Input: dimensioned drawing with shaded views. Units: mm. Origin: part minimum x, y, z. Round coordinates to 2 decimals unless told otherwise and drop trailing zeros. Order: outer loops, then holes, each group sorted by start corner. A loop starts at its lowest first (then second) coordinate and runs counter-clockwise, first axis right, second up.
Item 1: Cut plane B-B on y = 23. Output: boundary loops of the cut face in (x, z).
Item 2: Cut plane A-A on x = 13. Output: boundary loops of the cut face in (y, z), then the cut area to 3 significant figures.
Item 3: Cut plane C-C on z = 2.95. Output: boundary loops of the cut face in (x, y), then the cut area to 3 significant figures.
Item 4: Line query: L1, parallel to Y at x = 13, z = 2.85; L2, parallel to Y at x = 5, z = 3.2; L3, parallel to X at y = 16, z = 2.6. Output: solid intervals per line, ascending.
Item 5: First-contact query: pin 1 (4 mm diameter, centred on x = 21, y = 15, fed in from +Z); pin 2 (1.9 mm diameter, centred on x = 13, y = 23, fed in from -Z). Flat tips, straight axial feed; report the tip coordinate or a pass-through.
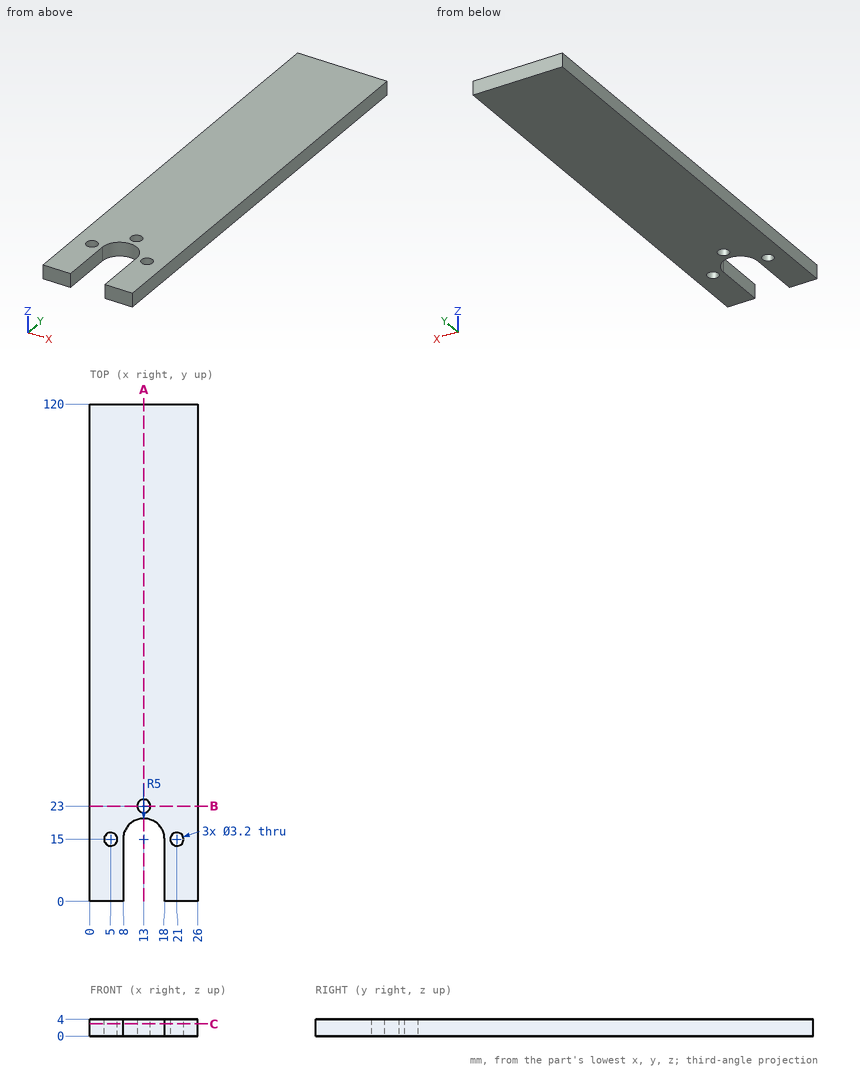
From the geometry:
1. outline: (0, 0) - (11.4, 0) - (11.4, 4) - (0, 4) - close; (14.6, 0) - (26, 0) - (26, 4) - (14.6, 4) - close
2. outline: (20, 0) - (21.4, 0) - (21.4, 4) - (20, 4) - close; (24.6, 0) - (120, 0) - (120, 4) - (24.6, 4) - close
2. area: 387 mm2
3. outline: (0, 0) - (8, 0) - (8, 15) arc R5 cw to (18, 15) - (18, 0) - (26, 0) - (26, 120) - (0, 120) - close; hole circle Ø3.2 at (5, 15); hole circle Ø3.2 at (13, 23); hole circle Ø3.2 at (21, 15)
3. area: 2,910 mm2
4. L1: y = 20 to 21.4, 24.6 to 120
4. L2: y = 0 to 13.4, 16.6 to 120
4. L3: x = 0 to 3.75, 6.25 to 8.1, 17.9 to 19.75, 22.25 to 26
5. pin 1: stops at z = 4
5. pin 2: passes through
